Geometry check sheet. Reference: the model listing, model coordinates, mm. Round coordinates to 2 decimals unless told otherwise and drop trailing zeros. Loops run counter-clockwise (first coordinate to the right, second up) from the corner with the lowest first, then second, coordinate; pieces in that order, holes last.
```python
from build123d import *

# Parameters (mm, degrees)
SKETCH002_W        = 112
SKETCH002_H        = 112
PAD001_DEPTH       = 5.5
SKETCH003_R        = 2.5
POCKET_DEPTH       = 322.475762
POLARPATTERN_COUNT = 4


with BuildPart() as part:
    # Sketch002 → Pad001 (new body)
    with BuildSketch(Plane.XZ):
        Rectangle(SKETCH002_W, SKETCH002_H)
    extrude(amount=-PAD001_DEPTH)

    # Sketch003 (on Face5 of Pad001) → Pocket (cut, through all)
    with BuildSketch(Plane.XZ):
        with Locations((-50, 50)):
            Circle(SKETCH003_R)
        with Locations((-37.5, 37.5)):
            Circle(SKETCH003_R)
    pocket = extrude(amount=-POCKET_DEPTH, mode=Mode.SUBTRACT)

    # PolarPattern: Pocket ×4 about axis
    polarpattern_axis = Axis((0, 0, 0), (0, -1, 0))
    for i in range(1, POLARPATTERN_COUNT):
        add(pocket.rotate(polarpattern_axis, i * 360 / POLARPATTERN_COUNT), mode=Mode.SUBTRACT)


solid = part.part
```
1) Gauge pin test, flat end, axial feed: pin 1 (4.5 mm diameter, centred on x = 50, z = 50, fed in from +Y). Record the tip position at first contact, or that the pin passes through.
Report:
pin 1: passes through
2) Mould release check, pull along X, two halves, no side actions. Record for faces 1 (the face through (56, 3, -1)), 2 (the face through (-1, 3, 56)), 3 (the face through (35.19, 2.71, -36.54)): +X half, -X half, draft (parallel to the pull), parting line (faces both ways), or undercut.
Report:
face 1: +X half
face 2: draft
face 3: undercut
3) Sectioned sample at B-B, the plane x = 37.5. Record the cut outline in (y, z).
Report:
outline: (0, -56) - (5.5, -56) - (5.5, -40) - (0, -40) - close; (0, -35) - (5.5, -35) - (5.5, 35) - (0, 35) - close; (0, 40) - (5.5, 40) - (5.5, 56) - (0, 56) - close
4) Sectioned sample at A-A, the plane z = -37.5. Record the cut outline in (x, y), then the cut area to 3 significant figures.
Report:
outline: (-56, 0) - (-40, 0) - (-40, 5.5) - (-56, 5.5) - close; (-35, 0) - (35, 0) - (35, 5.5) - (-35, 5.5) - close; (40, 0) - (56, 0) - (56, 5.5) - (40, 5.5) - close
area: 561 mm2
5) Scan lines: line 1 along Z through (x, y) = (-50, 2.2); line 2 along X through (y, z) = (3.2, -37.5). Record each from-to range of solid material in increasing order.
Report:
line 1: z = -56 to -52.5, -47.5 to 47.5, 52.5 to 56
line 2: x = -56 to -40, -35 to 35, 40 to 56
